Could you check a few things on this model? Use its own coordinates, in mm. Face numbers are marked on the shaded views. A direction names the side the tool comes from. Round coordinates to 2 decimals unless told otherwise and drop trailing zeros. Order: outer loops, then holes, each group sorted by start corner. A loop starts at its lowest first (then second) coordinate and runs counter-clockwise, first axis right, second up. Notation, with made-up numbers: M 14.25,40.5 L 33.25,40.5 A14 cw 33.25,52.5 Z; hole C 36,-3 d10. An arc over 180 degrees is marked long. Write each question's results on one line, items separated by ' | '. Start each with the question number.
1. Suppose I cut it at C-C on z = -60. Write out the boundary of the cut face in (x, y), and give its area (3 significant figures).
2. Please list where these lines run through material, in increasing order: L1, parallel to Z at x = 132, y = 31; L2, parallel to Z at x = -56.5, y = 109.5; L3, parallel to X at y = 28, z = 18.
3. Suppose I cut it at B-B on x = 136. Write out the boundary of the cut face in (y, z).
4. I'm going to push flat-ended pins straight in: pin 1 (12 mm diameter, centred on x = 126, y = 44, fed in from -Z); pin 2 (2 mm diameter, centred on x = 0, y = 33, fed in from -Z); pin 3 (1.5 mm diameter, centred on y = 33.5, z = -30.5, fed in from +X). Where does each tip first touch, or does it pass through?
5. For the marked faces 1 and 2, which set-ups out of +Z, -Z, +X, -X, +Y, -Y let a thin tool reach every point of the face, with its end or its side?
6. Suppose I cut it at A-A on y = 44. Write out the boundary of the cut face in (x, z), and give its area (3 significant figures).
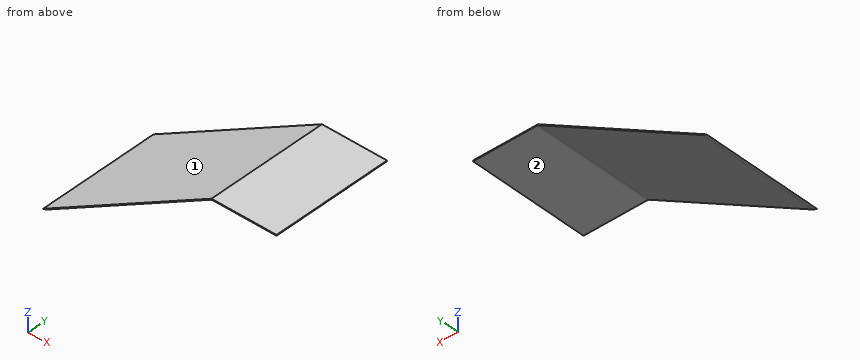
from build123d import *

# Parameters (mm, degrees)
EXTRUDE_1_DEPTH = 10
EXTRUDE_2_DEPTH = 150
FILLET_1_R      = 5
FILLET_2_R      = 5


with BuildPart() as part:
    # 草图1 → 凸台-拉伸1 (new body)
    with BuildSketch(Plane(origin=(0, 0, 0), x_dir=(1, 0, 0), z_dir=(0, 1, 0))):
        Polygon((-84.930519712, 76.342229186), (118.585450177, -41.157770814), (198.585450177, -41.157770814), (198.585450177, -42.157770814), (118.317500985, -42.157770814), (-89.528595923, 77.842229186), align=None)
    extrude(amount=EXTRUDE_1_DEPTH)

    # 草图1<2> → 凸台-拉伸2 (add)
    with BuildSketch(Plane(origin=(0, 0, 0), x_dir=(1, 0, 0), z_dir=(0, 1, 0))):
        Polygon((-84.930519712, 76.342229186), (118.585450177, -41.157770814), (198.585450177, -41.157770814), (198.585450177, -42.157770814), (118.317500985, -42.157770814), (-89.528595923, 77.842229186), align=None)
    extrude(amount=EXTRUDE_2_DEPTH)

    # 圆角1
    fillet_1_edges = [part.edges().sort_by_distance(p)[0] for p in [
        (-84.930519712, 75, -76.342229186),
    ]]
    fillet(fillet_1_edges, radius=FILLET_1_R)

    # 圆角2
    fillet_2_edges = [part.edges().sort_by_distance(p)[0] for p in [
        (118.585450177, 75, 41.157770814),
    ]]
    fillet(fillet_2_edges, radius=FILLET_2_R)


solid = part.part
Filled sheet:
1) outline: M -58.62,0 L -56.62,0 L -56.62,150 L -58.62,150 Z | area: 300 mm^2
2) L1: z = 41.16 to 42.16 | L2: z = -59.93 to -58.77 | L3: x = 76.48 to 78.48
3) outline: M 0,41.16 L 150,41.16 L 150,42.16 L 0,42.16 Z
4) pin 1: stops at z = 41.16 | pin 2: stops at z = -27.88 | pin 3: stops at x = -4.23
5) face 1: +Z, -X, +Y, -Y | face 2: -Z, +X, +Y, -Y
6) outline: M -89.53,-77.84 L -85.43,-76.5 A5 ccw -84.48,-76.08 L 117.43,40.49 A5 cw 119.93,41.16 L 198.59,41.16 L 198.59,42.16 L 118.32,42.16 Z | area: 318 mm^2
